The model under review builds one solid part; all positions refer to its coordinate system, in mm. Give positions to 0.01 mm unless a question says otherwise; leave off trailing zeros. Order: outer loops, then holes, each group sorted by start corner. A loop starts at its lowest first (then second) coordinate and runs counter-clockwise, first axis right, second up. Notation, with made-up numbers: (48, 1) - (74, 1) arc R23 ccw to (74, 28) - close; hole circle Ø8 at (-1, -4.5). An arc over 180 degrees is marked (long way). Use CSV: the item, a comma, the result in double quotes.
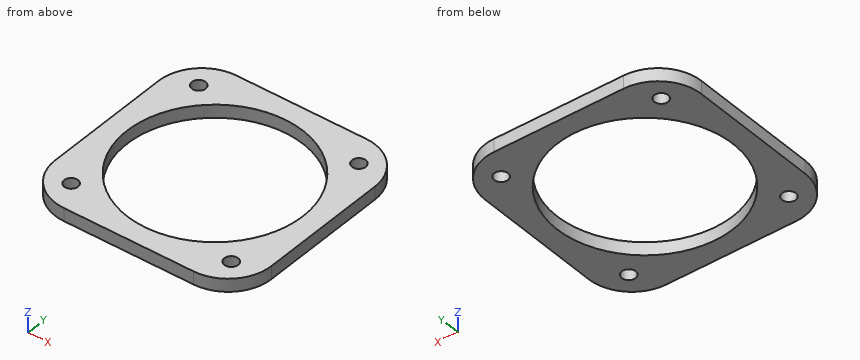
```python
from build123d import *

# Parameters (mm, degrees)
SKETCH_2_W      = 50
SKETCH_2_H      = 50
SKETCH_2_R      = 1.6
SKETCH_2_R_2    = 20.3
EXTRUDE_1_DEPTH = 3
FILLET_1_R      = 10


with BuildPart() as part:
    # 草图2 → 凸台-拉伸1 (new body)
    with BuildSketch(Plane.XY):
        Rectangle(SKETCH_2_W, SKETCH_2_H)
        with Locations((-18.5, 18.5)):
            Circle(SKETCH_2_R, mode=Mode.SUBTRACT)
        with Locations((18.5, 18.5)):
            Circle(SKETCH_2_R, mode=Mode.SUBTRACT)
        with Locations((18.5, -18.5)):
            Circle(SKETCH_2_R, mode=Mode.SUBTRACT)
        with Locations((-18.5, -18.5)):
            Circle(SKETCH_2_R, mode=Mode.SUBTRACT)
        Circle(SKETCH_2_R_2, mode=Mode.SUBTRACT)
    extrude(amount=EXTRUDE_1_DEPTH)

    # 圆角1
    fillet_1_edges = [part.edges().sort_by_distance(p)[0] for p in [
        (25, -25, 1.5),
        (-25, -25, 1.5),
        (-25, 25, 1.5),
        (25, 25, 1.5),
    ]]
    fillet(fillet_1_edges, radius=FILLET_1_R)


solid = part.part
```
Item 1: Take a section at C-C, the plane z = 0.95. Give the boundary of the cut face in (x, y).
Results list:
outline,"(-25, -15) arc R10 ccw to (-15, -25) - (15, -25) arc R10 ccw to (25, -15) - (25, 15) arc R10 ccw to (15, 25) - (-15, 25) arc R10 ccw to (-25, 15) - close; hole circle Ø40.6 at (0, 0); hole circle Ø3.2 at (-18.5, -18.5); hole circle Ø3.2 at (-18.5, 18.5); hole circle Ø3.2 at (18.5, -18.5); hole circle Ø3.2 at (18.5, 18.5)"
Item 2: Take a section at D-D, the plane x = -18.5. Give the boundary of the cut face in (y, z), and give its area (3 significant figures).
Results list:
outline,"(-24.37, 0) - (-20.1, 0) - (-20.1, 3) - (-24.37, 3) - close; (-16.9, 0) - (-8.36, 0) - (-8.36, 3) - (-16.9, 3) - close; (8.36, 0) - (16.9, 0) - (16.9, 3) - (8.36, 3) - close; (20.1, 0) - (24.37, 0) - (24.37, 3) - (20.1, 3) - close"
area,"76.9 mm2"
Item 3: Clearance check with a flat-ended pin moving along its axis: pin 1 (5 mm diameter, centred on x = -18.5, y = 18.5, fed in from +Z). State where the tip first meets the part, or that it passes through.
Results list:
pin 1,"stops at z = 3"
Item 4: Take a section at A-A, the plane x = 0. Give the boundary of the cut face in (y, z).
Results list:
outline,"(-25, 0) - (-20.3, 0) - (-20.3, 3) - (-25, 3) - close; (20.3, 0) - (25, 0) - (25, 3) - (20.3, 3) - close"
Item 5: Wall thickness on L1, parallel to Y at x = 0, z = 1.55; L2, parallel to Y at x = -18.5, z = 0.8; L3, parallel to Y at x = -4, z = 1.15: over which ranges is each line inside the solid? List them lowest first.
Results list:
L1,"y = -25 to -20.3, 20.3 to 25"
L2,"y = -24.37 to -20.1, -16.9 to -8.36, 8.36 to 16.9, 20.1 to 24.37"
L3,"y = -25 to -19.9, 19.9 to 25"
